Input: part model. Units: mm. Frame: model coordinates. Face numbers are marked on the shaded views. Give positions to 0.01 mm unless a question says otherwise; leave off trailing zeros. Loops run counter-clockwise (first coordinate to the right, second up) from the corner with the lowest first, then second, coordinate; pieces in that order, holes last. Notation, with made-up numbers: M -33,56 L -27,56 A10 cw -27,72 Z; hole C -18.75,57.25 d6. An arc over 180 degrees is marked long. Use CSV: the item, a comma, the result in double quotes. Start each with the question number.
from build123d import *

# Parameters (mm, degrees)
CROQUIS1_R                 = 29.72
CROQUIS1_R_2               = 25.4
SALIENTE_EXTRUIR1_DEPTH    = 250
CORTAR_EXTRUIR1_DEPTH      = 254.508494532
CORTAR_EXTRUIR1_DEPTH_BACK = 254.508494532
CROQUIS2_W                 = 3
CROQUIS2_H                 = 45


with BuildPart() as part:
    # Croquis1 → Saliente-Extruir1 (new body)
    with BuildSketch(Plane.XY):
        Circle(CROQUIS1_R)
        Circle(CROQUIS1_R_2, mode=Mode.SUBTRACT)
    extrude(amount=SALIENTE_EXTRUIR1_DEPTH)

    # Croquis2 → Cortar-Extruir1 (cut, two sides: drawn at the far end of the back side and taken through both)
    with BuildSketch(Plane(origin=(0, 0, 0), x_dir=(0, 0, -1), z_dir=(1, 0, 0)).offset(-CORTAR_EXTRUIR1_DEPTH_BACK)):
        with Locations((-193.5, 0)):
            Rectangle(CROQUIS2_W, CROQUIS2_H)
    extrude(amount=CORTAR_EXTRUIR1_DEPTH + CORTAR_EXTRUIR1_DEPTH_BACK, mode=Mode.SUBTRACT)


solid = part.part
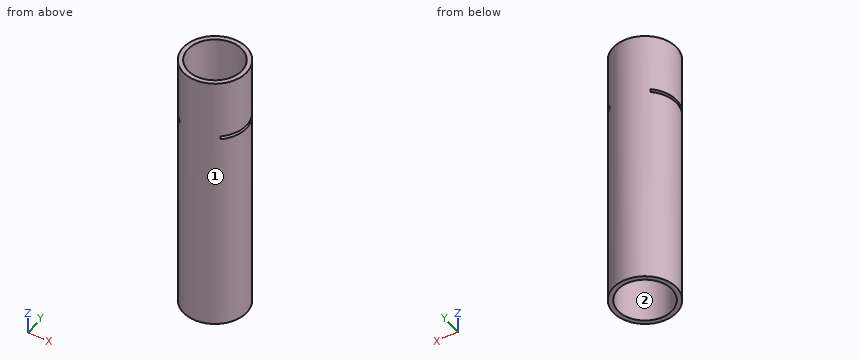
Item 1: Section A-A (y = 0). Output: boundary loops of the cut face in (x, z).
Item 2: Mould query, pull axis X, two halves, no side actions, for the marked faces 1 and 2. Classes: +X half, -X half, draft (parallel to the pull), parting line (faces both ways), or undercut.
Item 3: Material intervals for line 1 (Z direction, x = -15.5, y = -21); line 2 (X direction, y = 1, z = 57); line 3 (Y direction, x = 0, z = 145), sorted ascending.
Item 4: Section D-D (z = 59). Output: boundary loops of the cut face in (x, y), then the cut area to 3 significant figures.
Item 5: Section B-B (x = 0). Output: boundary loops of the cut face in (y, z), then the cut area to 3 significant figures.
Item 6: Section C-C (y = 19). Output: boundary loops of the cut face in (x, z).
Item 7: First-contact query: pin 1 Ø5.5 at (x, y) = (19, 7) entering from -Z; pin 2 Ø3 at (x, z) = (-5.5, 203.5) entering from -Y; pin 3 Ø12 at (x, y) = (-17, 17) entering from +Z; pin 4 Ø1.5 at (y, z) = (18, 136.5) entering from -X. Flat tips, straight axial feed; report the tip coordinate or a pass-through.
Recorded:
1,outline,"M -29.72,0 L -25.4,0 L -25.4,192 L -29.72,192 Z; M -29.72,195 L -25.4,195 L -25.4,250 L -29.72,250 Z; M 25.4,0 L 29.72,0 L 29.72,192 L 25.4,192 Z; M 25.4,195 L 29.72,195 L 29.72,250 L 25.4,250 Z"
2,face 1,"parting line"
2,face 2,"undercut"
3,line 1,"0 to 192, 195 to 250"
3,line 2,"-29.7 to -25.38, 25.38 to 29.7"
3,line 3,"-29.72 to -25.4, 25.4 to 29.72"
4,outline,"C 0,0 d59.44; hole C 0,0 d50.8"
4,area,"748 mm²"
5,outline,"M -29.72,0 L -25.4,0 L -25.4,250 L -29.72,250 Z; M 25.4,0 L 29.72,0 L 29.72,250 L 25.4,250 Z"
5,area,"2,160 mm²"
6,outline,"M -22.85,0 L -16.86,0 L -16.86,192 L -22.85,192 Z; M -22.85,195 L -16.86,195 L -16.86,250 L -22.85,250 Z; M 16.86,0 L 22.85,0 L 22.85,192 L 16.86,192 Z; M 16.86,195 L 22.85,195 L 22.85,250 L 16.86,250 Z"
7,pin 1,"through"
7,pin 2,"y = -29.45"
7,pin 3,"z = 250"
7,pin 4,"x = -24.2"
